from build123d import *

# Parameters (mm, degrees)
F3_DEPTH      = 15
F3_DEPTH_BACK = 65
F4_R          = 1.2
F5_DEPTH      = 124.25
F5_DEPTH_BACK = 109.5
F6_R          = 20
F8_DEPTH      = 2
F7_R          = 20
F9_DEPTH      = 2
F10_W         = 125.272244215
F10_H         = 20.9059882909
F11_DEPTH     = 40
F12_W         = 40
F12_H         = 22.6302481089
F13_DEPTH     = 10
F14_R         = 1
F15_DEPTH     = 50


with BuildPart() as f3:
    # F2 (on Front) → F3 (new body, two sides)
    with BuildSketch(Plane.XZ) as f3_sk:
        with BuildLine():
            Line((-30, 15), (-30, 0))
            Line((-30, 0), (30, 0))
            Line((30, 0), (30, 15))
            Line((30, 15), (23, 15))
            ThreePointArc((23, 15), (20.8786796564, 14.1213203436), (20, 12))
            Line((20, 12), (20, 3))
            Line((20, 3), (-20, 3))
            Line((-20, 3), (-20, 12))
            ThreePointArc((-20, 12), (-20.8786796564, 14.1213203436), (-23, 15))
            Line((-23, 15), (-30, 15))
        make_face()
    extrude(amount=F3_DEPTH)
    extrude(f3_sk.sketch, amount=-F3_DEPTH_BACK)

    # F4 (on face) → F5 (cut, two sides)
    with BuildSketch(Plane(origin=(0, 0, 0), x_dir=(1, 0, 0), z_dir=(0, -0.7071067812, 0.7071067812))) as f5_sk:
        with BuildLine():
            ThreePointArc((25.965, 0), (24.765, 1.2), (23.565, 0))
            ThreePointArc((23.565, 0), (24.765, -1.2), (25.965, 0))
        make_face()
        with Locations((-24.765, 0)):
            Circle(F4_R)
    extrude(amount=F5_DEPTH, mode=Mode.SUBTRACT)
    extrude(f5_sk.sketch, amount=-F5_DEPTH_BACK, mode=Mode.SUBTRACT)

    # F6 (on face) → F8 (join)
    with BuildSketch(Plane.YZ.offset(30)):
        with Locations((49.14, 7.5)):
            Circle(F6_R)
    extrude(amount=-F8_DEPTH)

    # F7 (on face) → F9 (join)
    with BuildSketch(Plane(origin=(-30, 0, 0), x_dir=(0, -1, 0), z_dir=(-1, 0, 0))):
        with Locations((-49.14, 7.5)):
            Circle(F7_R)
    extrude(amount=-F9_DEPTH)

    # F10 (on Right) → F11 (cut, symmetric)
    with BuildSketch(Plane.YZ):
        with Locations((62.6361221075, -10.4529941455)):
            Rectangle(F10_W, F10_H)
    extrude(amount=F11_DEPTH, both=True, mode=Mode.SUBTRACT)

    # F12 (on Top) → F13 (cut)
    with BuildSketch(Plane.XY):
        with Locations((0, 53.6848759456)):
            Rectangle(F12_W, F12_H)
    extrude(amount=F13_DEPTH, mode=Mode.SUBTRACT)

    # F14 (on Right) → F15 (cut, symmetric)
    with BuildSketch(Plane.YZ):
        with Locations((49.14, 7.5)):
            Circle(F14_R)
    extrude(amount=F15_DEPTH, both=True, mode=Mode.SUBTRACT)


solid = f3.part
Input: part model. Units: mm. Frame: model coordinates. A direction names the side the tool comes from. Give positions to 0.01 mm unless a question says otherwise; leave off trailing zeros. Write each loop counter-clockwise with the first axis right and the second up, starting at its lowest first coordinate (ties: lowest second). Pieces come first, ordered by that corner, then holes. Notation, with made-up numbers: (-6.75, -39) -> (8.25, -39) arc R29 cw to (8.25, -8) -> close; hole circle Ø5 at (10, 51.5). An arc over 180 degrees is marked (long way). Use one line per item in the form item = value. Start each with the question number.
1) Set-up query: faces 5 (the flat face through (0, 17, 0)), 6 (the cylindrical face through (-20.86, 24.44, 14.1)), 7 (the flat face through (26, 24, 15)), 8 (the flat face through (28, 54, 17)), 9 (the flat face through (-24, 65, 8)). Return all of +Z, -Z, +X, -X, +Y, -Y with unobstructed straight access to the full face (end or side cutting, diameter ignored); none if empty.
2) Section query A-A on y = 49.14. Return the cut outline in (x, z).
3) Ray query, probe 1 along Z at (x, y) = (-23.75, 49.14); probe 2 along X at (y, z) = (55.5, 25); probe 3 along Z at (x, y) = (-2.5, 20). Return the intervals inside material, ascending. Write a range as from..to.
4) Pin query (flat end, axial travel): pin 1 (2 mm diameter, centred on x = 26, y = 9, fed in from +Z); pin 2 (2 mm diameter, centred on x = -10, y = 2.5, fed in from +Z); pin 3 (9 mm diameter, centred on x = 23, z = 9, fed in from +Y). Return the tip coordinate at first contact, or that it passes through.
5) Section query B-B on z = 16.75. Return the cut outline in (x, y).
6) Section query C-C on z = 7.5. Count the separate pieces of the cut face and the enclosed holes in it, then the cut area to 3 significant figures.
7) Draft query along X for faces 1 (the flat face through (-30, 36, 11)), 2 (the flat face through (-26, 24, 15)), 3 (the flat face through (-20, 24, 7)), 4 (the cylindrical face through (29.01, 57.05, 25.87)). Return one class per face: pulls with the +X half, pulls with the -X half, needs draft (parallel to the pull), parting line crosses it, or undercut.
8) Section query D-D on y = 8. Return the cut outline in (x, z), then the cut area to 3 significant figures.
Outcome:
q1.face_5 = -Z, +X, -X, +Y, -Y
q1.face_6 = +Z, +Y, -Y
q1.face_7 = +Z, -Y
q1.face_8 = +Z, +Y
q1.face_9 = +Z, -Z, +Y
q2.outline = (-30, 0) -> (-20, 0) -> (-20, 6.5) -> (-30, 6.5) -> close; (-30, 8.5) -> (-20, 8.5) -> (-20, 12) arc R3 ccw to (-23, 15) -> (-28, 15) -> (-28, 27.5) -> (-30, 27.5) -> close; (20, 0) -> (30, 0) -> (30, 6.5) -> (20, 6.5) -> close; (20, 8.5) -> (30, 8.5) -> (30, 27.5) -> (28, 27.5) -> (28, 15) -> (23, 15) arc R3 ccw to (20, 12) -> close
q3.probe_1 = 0..6.5, 8.5..15
q3.probe_2 = -30..-28, 28..30
q3.probe_3 = 0..3
q4.pin_1 = 15
q4.pin_2 = 3
q4.pin_3 = 65
q5.outline = (-30, 31.41) -> (-28, 31.41) -> (-28, 66.87) -> (-30, 66.87) -> close; (28, 31.41) -> (30, 31.41) -> (30, 66.87) -> (28, 66.87) -> close
q6.separate_pieces = 4
q6.enclosed_holes = 2
q6.area = 1,560 mm^2
q7.face_1 = pulls with the -X half
q7.face_2 = undercut
q7.face_3 = undercut
q7.face_4 = needs draft
q8.outline = (-30, 0) -> (30, 0) -> (30, 15) -> (23, 15) arc R3 ccw to (20, 12) -> (20, 3) -> (-20, 3) -> (-20, 12) arc R3 ccw to (-23, 15) -> (-30, 15) -> close
q8.area = 416 mm^2
